from build123d import *

# Parameters (mm, degrees)
FILLET1_R          = 6
SKETCH2_R          = 3
CUT_EXTRUDE1_DEPTH = 51


with BuildPart() as part:
    # Sketch1 → Revolve1 (revolve)
    with BuildSketch(Plane.XY):
        Polygon((0, 22.5), (-20, 22.5), (-20, 25.25), (-23, 25.25), (-23, 25), (-47, 25), (-47, 25.25), (-53, 25.25), (-53, 37.5), (-23, 37.5), (-23, 80), (-3, 80), (-3, 60), (0, 60), align=None)
    revolve(axis=Axis((-1000, 0, 0), (1, 0, 0)))

    # Fillet1
    fillet1_edges = [part.edges().sort_by_distance(p)[0] for p in [
        (-23, -37.5, 0),
    ]]
    fillet(fillet1_edges, radius=FILLET1_R)

    # Sketch2 → Cut-Extrude1 (cut, through all)
    with BuildSketch(Plane(origin=(-3, 0, 0), x_dir=(0, 0, -1), z_dir=(1, 0, 0))):
        with Locations((0, 70)):
            Circle(SKETCH2_R)
        with Locations((60.621778265, -35)):
            Circle(SKETCH2_R)
        with Locations((-60.621778265, -35)):
            Circle(SKETCH2_R)
    extrude(amount=-CUT_EXTRUDE1_DEPTH, mode=Mode.SUBTRACT)


solid = part.part
Can you work these out from the model? Positions are in its coordinate system, mm. A direction names the side the tool comes from. Coordinates: 2 decimals unless noted, no trailing zeros. Loops run counter-clockwise (first coordinate to the right, second up) from the corner with the lowest first, then second, coordinate; pieces in that order, holes last. Notation, with made-up numbers: M 39,7 L 47,7 A18 ccw 47,26 Z; hole C 33.25,-6 d2. An arc over 180 degrees is marked long. Return JSON: item names as keys, results as strings. Group by question number.
Item 1: Thinking about a two-plate mould opening in Y: for faces 1 (the flat face through (-20, 17, -15)), 2 (the cylindrical face through (-12.86, -17.34, -78.1)), 3 (the flat face through (-23, -34, -34)), which applies, released by +Y, released by -Y, zero draft, split by the parting line, or undercut?
Item 2: Imagine slicing it at B-B (z = 0). Give the number of separate pieces and of enclosed holes in the cut face, and give its area (3 significant figures).
Item 3: Imagine slicing it at C-C (x = -10.5). Please give me the cut outline in (y, z), and give its area (3 significant figures).
Item 4: Imagine slicing it at D-D (x = -40). Please give me the cut outline in (y, z), and give its area (3 significant figures).
Item 5: I'm going to push flat-ended pins straight in: pin 1 Ø1 at (y, z) = (-10, -49.5) entering from -X; pin 2 Ø5.5 at (y, z) = (-35, -60.62) entering from -X; pin 3 Ø12 at (x, y) = (-35, 30.5) entering from -Z; pin 4 Ø8 at (x, y) = (-12, -15.5) entering from -Z. Where does each tip first touch, or does it pass through?
Item 6: If I drill on L1, parallel to Z at x = -18, y = -33; L2, parallel to X at y = 50, z = -19.5; L3, parallel to X at y = 50, z = -56.5, over which ranges is the centre line in solid material (lowest first)? Write a range as from..to.
Item 7: On a 3-axis mill with a long thin cutter (end or side, diameter ignored), from which of +Z, -Z, +X, -X, +Y, -Y can I reach the whole of each face in a straight line? I mean faces 4 (the flat face through (-53, -24.5, -7.8)), 5 (the cylindrical face through (-21.52, -5.47, -24.65)), 6 (the flat face through (0, -1, -26)), 7 (the cylindrical face through (-40.83, -4.88, 37.18)), 8 (the cylindrical face through (-1.48, -59.94, 2.64)). Say none if no direction works.
Verdict:
{
 "1": {"face 1": "undercut", "face 2": "split by the parting line", "face 3": "zero draft"},
 "2": {"separate pieces": "3", "enclosed holes": "0", "area": "3,150 mm^2"},
 "3": {"outline": "C 0,0 d160; hole C -35,-60.62 d6; hole C -35,60.62 d6; hole C 0,0 d45; hole C 70,0 d6", "area": "18,400 mm^2"},
 "4": {"outline": "C 0,0 d75; hole C 0,0 d50", "area": "2,450 mm^2"},
 "5": {"pin 1": "stops at x = -23", "pin 2": "passes through", "pin 3": "stops at z = -28.39", "pin 4": "stops at z = -79.17"},
 "6": {"L1": "z = -72.88..-62.86, -58.39..58.39, 62.86..72.88", "L2": "x = -23..0", "L3": "x = -23..-3"},
 "7": {"face 4": "+Z, -Z, -X, +Y, -Y", "face 5": "none", "face 6": "+Z, -Z, +X, +Y, -Y", "face 7": "-X", "face 8": "+X"}
}
